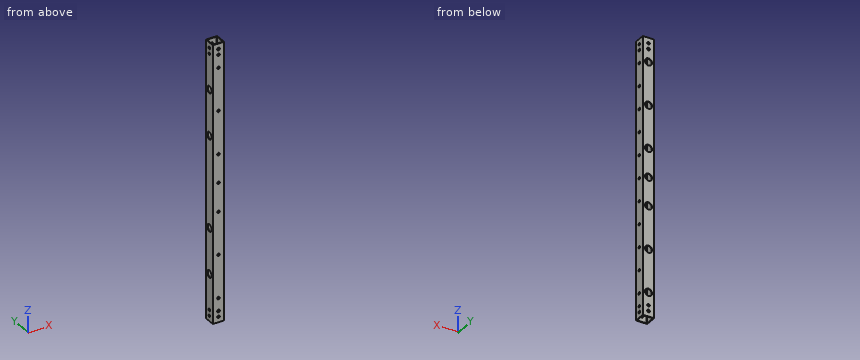
from build123d import *

# Parameters (mm, degrees)
CROQUIS1_W              = 20
CROQUIS1_H              = 20
CROQUIS1_W_2            = 17.4
CROQUIS1_H_2            = 17.4
SALIENTE_EXTRUIR2_DEPTH = 242
FILLET1_R               = 0.75
SKETCH1_R               = 2.35
CUT_EXTRUDE1_DEPTH      = 244.030862238
SKETCH2_R               = 2.25
CUT_EXTRUDE4_DEPTH      = 244.030862238
SKETCH2_5_R             = 6.3
SKETCH2_5_R_2           = 2.25
CUT_EXTRUDE5_DEPTH      = 5
SKETCH3_R               = 2.25
CUT_EXTRUDE6_DEPTH      = 5
SKETCH4_R               = 6.3
CUT_EXTRUDE7_DEPTH      = 5
SKETCH3_2_R             = 2.25
CUT_EXTRUDE8_DEPTH      = 244.030862238


with BuildPart() as part:
    # Croquis1 → Saliente-Extruir2 (new, symmetric)
    with BuildSketch(Plane.XY):
        Rectangle(CROQUIS1_W, CROQUIS1_H)
        Rectangle(CROQUIS1_W_2, CROQUIS1_H_2, mode=Mode.SUBTRACT)
    extrude(amount=SALIENTE_EXTRUIR2_DEPTH, both=True)

    # Fillet1
    fillet1_edges = [part.edges().sort_by_distance(p)[0] for p in [
        (-8.7, 8.7, 0),
        (-8.7, -8.7, 0),
        (8.7, -8.7, 0),
        (8.7, 8.7, 0),
    ]]
    fillet(fillet1_edges, radius=FILLET1_R)

    # Sketch1 → Cut-Extrude1 (cut, through all)
    with BuildSketch(Plane(origin=(0, 10, 0), x_dir=(1, 0, 0), z_dir=(0, 1, 0))):
        with Locations(Location((0, -232.5, 0), (0, 0, 270))):
            Circle(SKETCH1_R)
        with Locations(Location((0, -222.5, 0), (0, 0, 270))):
            Circle(SKETCH1_R)
        with Locations(Location((0, 222.5, 0), (0, 0, 270))):
            Circle(SKETCH1_R)
        with Locations(Location((0, 232.5, 0), (0, 0, 270))):
            Circle(SKETCH1_R)
    extrude(amount=-CUT_EXTRUDE1_DEPTH, mode=Mode.SUBTRACT)

    # Sketch2 → Cut-Extrude4 (cut, through all)
    with BuildSketch(Plane(origin=(0, 10, 0), x_dir=(0, 0, -1), z_dir=(0, -1, 0))):
        with Locations(Location((200, 0, 0), (0, 0, 180))):
            Circle(SKETCH2_R)
        with Locations((-200, 0)):
            Circle(SKETCH2_R)
        with Locations((-125, 0)):
            Circle(SKETCH2_R)
        with Locations((-50, 0)):
            Circle(SKETCH2_R)
        Circle(SKETCH2_R)
        with Locations((50, 0)):
            Circle(SKETCH2_R)
        with Locations((125, 0)):
            Circle(SKETCH2_R)
    extrude(amount=CUT_EXTRUDE4_DEPTH, mode=Mode.SUBTRACT)

    # Sketch2<5> → Cut-Extrude5 (cut)
    # profile 1 of 7: a face of its own
    with BuildSketch(Plane(origin=(0, 10, 0), x_dir=(0, 0, -1), z_dir=(0, -1, 0))):
        with Locations(Location((-125, 0, 0), (0, 0, 180))):
            Circle(SKETCH2_5_R)
        with Locations(Location((-125, 0, 0), (0, 0, 180))):
            Circle(SKETCH2_5_R_2, mode=Mode.SUBTRACT)
    # profile 2 of 7: a face of its own
    with BuildSketch(Plane(origin=(0, 10, 0), x_dir=(0, 0, -1), z_dir=(0, -1, 0))):
        with Locations((-200, 0)):
            Circle(SKETCH2_5_R)
    # profile 3 of 7: a face of its own
    with BuildSketch(Plane(origin=(0, 10, 0), x_dir=(0, 0, -1), z_dir=(0, -1, 0))):
        with Locations((-50, 0)):
            Circle(SKETCH2_5_R)
    # profile 4 of 7: a face of its own
    with BuildSketch(Plane(origin=(0, 10, 0), x_dir=(0, 0, -1), z_dir=(0, -1, 0))):
        Circle(SKETCH2_5_R)
    # profile 5 of 7: a face of its own
    with BuildSketch(Plane(origin=(0, 10, 0), x_dir=(0, 0, -1), z_dir=(0, -1, 0))):
        with Locations((50, 0)):
            Circle(SKETCH2_5_R)
    # profile 6 of 7: a face of its own
    with BuildSketch(Plane(origin=(0, 10, 0), x_dir=(0, 0, -1), z_dir=(0, -1, 0))):
        with Locations((125, 0)):
            Circle(SKETCH2_5_R)
    # profile 7 of 7: a face of its own
    with BuildSketch(Plane(origin=(0, 10, 0), x_dir=(0, 0, -1), z_dir=(0, -1, 0))):
        with Locations((200, 0)):
            Circle(SKETCH2_5_R)
    extrude(amount=CUT_EXTRUDE5_DEPTH, mode=Mode.SUBTRACT)

    # Sketch3 → Cut-Extrude6 (cut)
    with BuildSketch(Plane.ZY.offset(-10)):
        Circle(SKETCH3_R)
        with Locations((40, 0)):
            Circle(SKETCH3_R)
        with Locations((80, 0)):
            Circle(SKETCH3_R)
        with Locations((120, 0)):
            Circle(SKETCH3_R)
        with Locations((160, 0)):
            Circle(SKETCH3_R)
        with Locations((-40, 0)):
            Circle(SKETCH3_R)
        with Locations((-80, 0)):
            Circle(SKETCH3_R)
        with Locations((-120, 0)):
            Circle(SKETCH3_R)
        with Locations((-160, 0)):
            Circle(SKETCH3_R)
        with Locations((-200, 0)):
            Circle(SKETCH3_R)
        with Locations((200, 0)):
            Circle(SKETCH3_R)
        with Locations((-232.5, 0)):
            Circle(SKETCH3_R)
        with Locations((-222.5, 0)):
            Circle(SKETCH3_R)
        with Locations((232.5, 0)):
            Circle(SKETCH3_R)
        with Locations((222.5, 0)):
            Circle(SKETCH3_R)
    extrude(amount=CUT_EXTRUDE6_DEPTH, mode=Mode.SUBTRACT)

    # Sketch4 → Cut-Extrude7 (cut)
    with BuildSketch(Plane.ZY.offset(10)):
        with Locations(Location((-160, 0, 0), (0, 0, 270))):
            Circle(SKETCH4_R)
        with Locations(Location((-80, 0, 0), (0, 0, 270))):
            Circle(SKETCH4_R)
        with Locations(Location((80, 0, 0), (0, 0, 270))):
            Circle(SKETCH4_R)
        with Locations(Location((160, 0, 0), (0, 0, 270))):
            Circle(SKETCH4_R)
    extrude(amount=-CUT_EXTRUDE7_DEPTH, mode=Mode.SUBTRACT)

    # Sketch3<2> → Cut-Extrude8 (cut, through all)
    with BuildSketch(Plane.ZY.offset(-10)):
        with Locations((-232.5, 0)):
            Circle(SKETCH3_2_R)
        with Locations((-222.5, 0)):
            Circle(SKETCH3_2_R)
        with Locations((232.5, 0)):
            Circle(SKETCH3_2_R)
        with Locations((222.5, 0)):
            Circle(SKETCH3_2_R)
    extrude(amount=CUT_EXTRUDE8_DEPTH, mode=Mode.SUBTRACT)


solid = part.part
Here's how the part is built. I have some questions about the finished solid (model axes, mm). Round coordinates to 2 decimals unless told otherwise and drop trailing zeros. Order: outer loops, then holes, each group sorted by start corner. A loop starts at its lowest first (then second) coordinate and runs counter-clockwise, first axis right, second up. Notation, with made-up numbers: M 28,65.5 L 33,65.5 A13 cw 33,74.5 Z; hole C 4.5,87 d4. An arc over 180 degrees is marked long. Return JSON: item names as keys, results as strings. Group by question number.
1. I'm going to push flat-ended pins straight in: pin 1 Ø11.5 at (x, z) = (0, 125) entering from +Y; pin 2 Ø7 at (y, z) = (0, 80) entering from -X; pin 3 Ø4 at (x, z) = (0, -232.5) entering from -Y; pin 4 Ø2.5 at (y, z) = (0, 200) entering from +X. Where does each tip first touch, or does it pass through?
2. If we section it at A-A on z = 172: List the corners of the cut face in (x, y) for me, then the cut area to 3 significant figures.
3. Please list where these lines run through material, in increasing order: probe 1 along X at (y, z) = (8, -117.5); probe 2 along X at (y, z) = (9.3, 200).
Reply:
{
 "1": {"pin 1": "y = -8.7", "pin 2": "x = 8.7", "pin 3": "through", "pin 4": "x = -8.7"},
 "2": {"outline": "M -10,-10 L 10,-10 L 10,10 L -10,10 Z; hole M -8.7,-7.95 A0.75 ccw -7.95,-8.7 L 7.95,-8.7 A0.75 ccw 8.7,-7.95 L 8.7,7.95 A0.75 ccw 7.95,8.7 L -7.95,8.7 A0.75 ccw -8.7,7.95 Z", "area": "97.7 mm^2"},
 "3": {"probe 1": "-10 to -8.7, 8.7 to 10", "probe 2": "-10 to -6.3, 6.3 to 10"}
}
